from build123d import *

# Parameters (mm, degrees)
SKETCH1_R           = 5
BOSS_EXTRUDE1_DEPTH = 25
SKETCH2_R           = 10
CUT_EXTRUDE1_DEPTH  = 50
SCALE1_SCALE        = 0.3


with BuildPart() as part:
    # Sketch1 → Boss-Extrude1 (new body, symmetric)
    with BuildSketch(Plane.XY):
        with BuildLine():
            Line((150, 25), (160, 25))
            ThreePointArc((160, 25), (174.142135624, 19.142135624), (180, 5))
            Line((180, 5), (180, -125))
            Line((180, -125), (130, -125))
            Line((130, -125), (130, 5))
            ThreePointArc((130, 5), (135.857864376, 19.142135624), (150, 25))
        make_face()
        with Locations((150, 5)):
            Circle(SKETCH1_R, mode=Mode.SUBTRACT)
    extrude(amount=BOSS_EXTRUDE1_DEPTH, both=True)

    # Sketch2 → Cut-Extrude1 (cut)
    with BuildSketch(Plane.XZ.offset(125)):
        with Locations((155, 0)):
            Circle(SKETCH2_R)
    extrude(amount=-CUT_EXTRUDE1_DEPTH, mode=Mode.SUBTRACT)


with BuildPart() as part_1:
    # Scale1: scaled about (155.056620621, -50.103937956, 0)
    add(part.part.scale(SCALE1_SCALE).moved(Location((108.539634435, -35.072756569, 0))))


solid = part_1.part
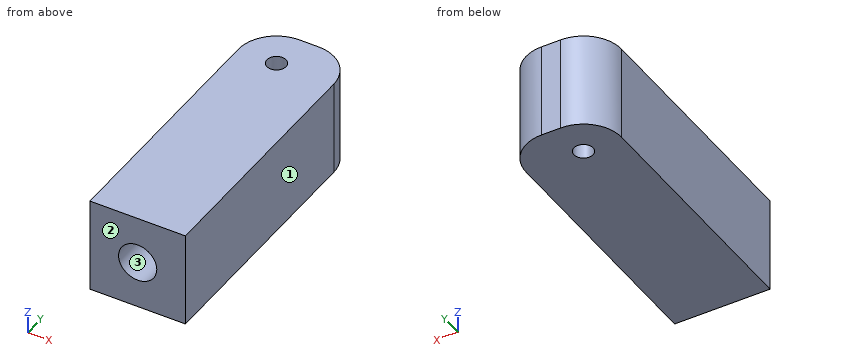
The model under review builds one solid part; all positions refer to its coordinate system, in mm. Face numbers are marked on the shaded views. Round coordinates to 2 decimals unless told otherwise and drop trailing zeros. Order: outer loops, then holes, each group sorted by start corner. A loop starts at its lowest first (then second) coordinate and runs counter-clockwise, first axis right, second up. Notation, with made-up numbers: (37, 45.25) -> (81, 45.25) arc R15 cw to (81, 51.25) -> close; hole circle Ø11 at (27, -23). An arc over 180 degrees is marked (long way). Use CSV: the item, a comma, the result in double quotes. Start each with the question number.
(1) Consider section D-D on z = 0. Write out the cut boundary in (x, y), and give its area (3 significant figures).
(2) Insertion check: pin 1 (3 mm diameter, centred on x = 155.5, z = 0.5, fed in from -Y); pin 2 (1 mm diameter, centred on x = 150, z = 1, fed in from +Y); pin 3 (6 mm diameter, centred on x = 160, z = 3, fed in from +Y). Each pin has a flat end and moves straight along its axis. Give the tip position at first contact, or say it passes through.
(3) Consider section B-B on x = 154. Write out the cut boundary in (y, z).
(4) Consider section A-A on z = 3.75. Write out the cut boundary in (x, y).
(5) Consider section C-C on y = -34. Write out the cut boundary in (x, z), and give its area (3 significant figures).
(6) Mouldability with a two-part tool opening along X and no side actions: class the marked faces 1, 2 and 3 as pulls with the +X half, pulls with the -X half, needs draft (parallel to the pull), parting line crosses it, or undercut.
(7) Wall thickness on probe 1 along Y at (x, z) = (153.5, 1.5); probe 2 along Y at (x, z) = (153, 6.5); probe 3 along Y at (x, z) = (156.75, 3.5): over which ranges is each line inside the solid? List them lowest first. Write a range as from..to.
Responses:
1,outline,"(147.54, -72.57) -> (152.04, -72.57) -> (152.04, -57.57) -> (158.04, -57.57) -> (158.04, -72.57) -> (162.54, -72.57) -> (162.54, -33.57) arc R6 ccw to (156.54, -27.57) -> (153.54, -27.57) arc R6 ccw to (147.54, -33.57) -> close; hole circle Ø3 at (153.54, -33.57)"
1,area,"562 mm²"
2,pin 1,"y = -57.57"
2,pin 2,"y = -28.4"
2,pin 3,"y = -27.59"
3,outline,"(-72.57, -7.5) -> (-35, -7.5) -> (-35, 7.5) -> (-72.57, 7.5) -> (-72.57, 2.81) -> (-57.57, 2.81) -> (-57.57, -2.81) -> (-72.57, -2.81) -> close; (-32.15, -7.5) -> (-27.57, -7.5) -> (-27.57, 7.5) -> (-32.15, 7.5) -> close"
4,outline,"(147.54, -72.57) -> (162.54, -72.57) -> (162.54, -33.57) arc R6 ccw to (156.54, -27.57) -> (153.54, -27.57) arc R6 ccw to (147.54, -33.57) -> close; hole circle Ø3 at (153.54, -33.57)"
5,outline,"(147.54, -7.5) -> (152.1, -7.5) -> (152.1, 7.5) -> (147.54, 7.5) -> close; (154.98, -7.5) -> (162.54, -7.5) -> (162.54, 7.5) -> (154.98, 7.5) -> close"
5,area,"182 mm²"
6,face 1,"pulls with the +X half"
6,face 2,"needs draft"
6,face 3,"undercut"
7,probe 1,"-57.57..-35.07, -32.07..-27.57"
7,probe 2,"-72.57..-34.97, -32.17..-27.6"
7,probe 3,"-72.57..-27.58"
